Build history of the part. All positions in model axes, mm. A direction names the side the tool comes from. Round coordinates to 2 decimals unless told otherwise and drop trailing zeros. Write each loop counter-clockwise with the first axis right and the second up, starting at its lowest first coordinate (ties: lowest second). Pieces come first, ordered by that corner, then holes. Notation, with made-up numbers: (83, 53) - (125, 53) arc R23 cw to (125, 74) - close; hole circle Ø3 at (58.5, 40.5). An arc over 180 degrees is marked (long way). One line per question, with ' | ' between items.
from build123d import *


with BuildPart() as part:
    # 草图1 → 旋转1 (revolve)
    with BuildSketch(Plane.XY, mode=Mode.PRIVATE) as revolve_1_sk:
        with BuildLine():
            Line((0, 56), (0, -25))
            Line((0, -25), (19.5, -25))
            ThreePointArc((19.5, -25), (22.328427125, -23.828427125), (23.5, -21))
            Line((23.5, -21), (23.5, 25))
            Line((23.5, 25), (23.5, 28))
            ThreePointArc((23.5, 28), (20.863961031, 34.363961031), (14.5, 37))
            Line((14.5, 37), (14.5, 42))
            Line((14.5, 42), (15.90903206, 42))
            Line((15.90903206, 42), (15.90903206, 44))
            Line((15.90903206, 44), (15.5, 44))
            Line((15.5, 44), (15.5, 56))
            Line((15.5, 56), (0, 56))
        make_face()
    revolve(revolve_1_sk.sketch.rotate(Axis((0, 0, 0), (0, 1, 0)), 90), axis=Axis((0, 0, 0), (0, 1, 0)))


solid = part.part
Q1. Saw through at C-C, the plane y = 24. List the corners of the cut face in (x, z).
Found:
outline: circle Ø47 at (0, 0)
Q2. Saw through at B-B, the plane z = 0. List the corners of the cut face in (x, y).
Found:
outline: (-23.5, -21) arc R4 ccw to (-19.5, -25) - (19.5, -25) arc R4 ccw to (23.5, -21) - (23.5, 28) arc R9 ccw to (14.5, 37) - (14.5, 42) - (15.91, 42) - (15.91, 44) - (15.5, 44) - (15.5, 56) - (-15.5, 56) - (-15.5, 44) - (-15.91, 44) - (-15.91, 42) - (-14.5, 42) - (-14.5, 37) arc R9 ccw to (-23.5, 28) - close
Q3. Pull direction Y, two halves, no side cores. Call faces 4 (the cylindrical face through (12.864, 39.535, -6.691)), 5 (the flat face through (0, 56, 0)), 6 (the cylindrical face through (-15.368, 50.084, 2.018)): +Y half, -Y half, draft (parallel to the pull), parting line (faces both ways), or undercut.
Found:
face 4: undercut | face 5: +Y half | face 6: draft
Q4. Which spindle directions (+Z, -Z, +X, -X, +Y, -Y) get a long thin tool onto all of the face, cutting with end or side? Do faces 1 (the cylindrical face through (9.68, 43.014, 12.625)), 2 (the flat face through (7, 42, 13)), 3 (the flat face through (0, -25, 0)). Say none if no direction does.
Found:
face 1: +Y | face 2: none | face 3: +Z, -Z, +X, -X, -Y
Q5. Drill centre lines: L1, parallel to Z at x = -16, y = 10; L2, parallel to X at y = -7, z = 20.5; L3, parallel to X at y = -12, z = -17. Where is each one in solid material? Low to high. Write a range as from..to.
Found:
L1: -17.21..17.21 | L2: -11.49..11.49 | L3: -16.22..16.22
Q6. Saw through at D-D, the plane y = 34. List the corners of the cut face in (x, z), then the cut area to 3 significant figures.
Found:
outline: circle Ø42.42 at (0, 0) | area: 1,410 mm^2
Q7. Drop flat-ended pins along their axis: pin 1 (4 mm diameter, centred on y = -10, z = -15, fed in from -X); pin 2 (6 mm diameter, centred on x = 6.5, z = -18, fed in from +Y); pin 3 (12 mm diameter, centred on y = -3, z = -14, fed in from -X). Give the stop position or say it passes through.
Found:
pin 1: x = -19.58 | pin 2: y = 36.85 | pin 3: x = -22.1
Q8. Saw through at A-A, the plane x = 0. List the corners of the cut face in (y, z).
Found:
outline: (-25, -19.5) arc R4 ccw to (-21, -23.5) - (28, -23.5) arc R9 ccw to (37, -14.5) - (42, -14.5) - (42, -15.91) - (44, -15.91) - (44, -15.5) - (56, -15.5) - (56, 15.5) - (44, 15.5) - (44, 15.91) - (42, 15.91) - (42, 14.5) - (37, 14.5) arc R9 ccw to (28, 23.5) - (-21, 23.5) arc R4 ccw to (-25, 19.5) - close
